```python
from build123d import *

# Parameters (mm, degrees)
PAD004_DEPTH    = 50
PAD003_DEPTH    = 50
BOX001_W        = 33
BOX001_H        = 20
BOX001_DEPTH    = 51
BOX_W           = 33
BOX_H           = 20
BOX_DEPTH       = 51
BOX002_W        = 33
BOX002_H        = 20
BOX002_DEPTH    = 51
BOX003_W        = 33
BOX003_H        = 20
BOX003_DEPTH    = 51
SKETCH_R        = 25
PAD_DEPTH       = 30
PAD002_DEPTH    = 50
SKETCH001_R     = 40
PAD001_DEPTH    = 75
SKETCH005_W     = 21.319589
SKETCH005_H     = 49.375387
POCKET_DEPTH    = 0.2
SKETCH006_R     = 15
POCKET001_DEPTH = 43.555516


with BuildPart() as pad004:
    # Sketch004 → Pad004 (new body, symmetric)
    with BuildSketch(Plane.XZ):
        Polygon((-40, 70), (-20, 104.849875), (-40, 104.849875), align=None)
    extrude(amount=PAD004_DEPTH, both=True)


with BuildPart() as pad003:
    # Sketch003 → Pad003 (new body, symmetric)
    with BuildSketch(Plane.XZ):
        Polygon((20, 105), (40, 69.438118), (40, 105), align=None)
    extrude(amount=PAD003_DEPTH, both=True)


with BuildPart() as cubo001:
    # Box001 → Box001 (new body)
    with BuildSketch(Plane(origin=(5, -40, 55), x_dir=(1, 0, 0), z_dir=(0, 0, 1))):
        with Locations((16.5, 10)):
            Rectangle(BOX001_W, BOX001_H)
    extrude(amount=BOX001_DEPTH)


with BuildPart() as cubo:
    # Box → Box (new body)
    with BuildSketch(Plane(origin=(5, 20, 55), x_dir=(1, 0, 0), z_dir=(0, 0, 1))):
        with Locations((16.5, 10)):
            Rectangle(BOX_W, BOX_H)
    extrude(amount=BOX_DEPTH)


with BuildPart() as cubo002:
    # Box002 → Box002 (new body)
    with BuildSketch(Plane(origin=(-38, -40, 55), x_dir=(1, 0, 0), z_dir=(0, 0, 1))):
        with Locations((16.5, 10)):
            Rectangle(BOX002_W, BOX002_H)
    extrude(amount=BOX002_DEPTH)


with BuildPart() as cubo003:
    # Box003 → Box003 (new body)
    with BuildSketch(Plane(origin=(-38, 20, 55), x_dir=(1, 0, 0), z_dir=(0, 0, 1))):
        with Locations((16.5, 10)):
            Rectangle(BOX003_W, BOX003_H)
    extrude(amount=BOX003_DEPTH)


with BuildPart() as pad:
    # Sketch → Pad (new body)
    with BuildSketch(Plane.XY):
        Circle(SKETCH_R)
    extrude(amount=PAD_DEPTH)


with BuildPart() as pad002:
    # Sketch002 → Pad002 (new body, symmetric)
    with BuildSketch(Plane(origin=(-81, 0, 6), x_dir=(1, 0, 0), z_dir=(0, -1, 0))):
        with BuildLine():
            Line((61.374028, 37.554516), (102.260882, 37.554516))
            Line((102.260882, 37.554516), (102.260882, 66.257331))
            ThreePointArc((102.260882, 66.257331), (98.26163, 79.156523), (87.211113, 86.919851))
            Line((87.211113, 86.919851), (87.11186, 102.554516))
            Line((87.11186, 102.554516), (75.11186, 102.554516))
            Line((75.11186, 102.554516), (75.158353, 85.860966))
            ThreePointArc((75.158353, 85.860966), (65.381997, 78.874221), (61.374028, 67.54603))
            Line((61.374028, 37.554516), (61.374028, 67.54603))
        make_face()
    extrude(amount=PAD002_DEPTH, both=True)


with BuildPart() as pocket001:
    # Pad001 base: copy of Pad
    add(pad.part)

    # Sketch001 → Pad001 (new body)
    with BuildSketch(Plane.XY.offset(30)):
        Circle(SKETCH001_R)
    extrude(amount=PAD001_DEPTH)

    # Cut: cut Pad002
    add(pad002.part, mode=Mode.SUBTRACT)

    # Fusion: union Pad
    add(pad.part)

    # Cut001: cut Cubo003
    add(cubo003.part, mode=Mode.SUBTRACT)

    # Cut002: cut Cubo002
    add(cubo002.part, mode=Mode.SUBTRACT)

    # Cut003: cut Cubo
    add(cubo.part, mode=Mode.SUBTRACT)

    # Cut004: cut Cubo001
    add(cubo001.part, mode=Mode.SUBTRACT)

    # Cut005: cut Pad003
    add(pad003.part, mode=Mode.SUBTRACT)

    # Cut006: cut Pad004
    add(pad004.part, mode=Mode.SUBTRACT)

    # Sketch005 → Pocket (cut)
    with BuildSketch(Plane.XY.offset(105)):
        with Locations((-30.63901, -1.115778)):
            Rectangle(SKETCH005_W, SKETCH005_H)
    extrude(amount=-POCKET_DEPTH, mode=Mode.SUBTRACT)

    # Sketch006 → Pocket001 (cut, through all)
    with BuildSketch(Plane.XY.offset(43.554516)):
        Circle(SKETCH006_R)
    extrude(amount=-POCKET001_DEPTH, mode=Mode.SUBTRACT)


solid = pocket001.part
```
Model file for the job. Use its own axes, mm. A direction names the side the tool comes from. Round coordinates to 2 decimals unless told otherwise and drop trailing zeros. Write each loop counter-clockwise with the first axis right and the second up, starting at its lowest first coordinate (ties: lowest second). Pieces come first, ordered by that corner, then holes. Notation, with made-up numbers: (17, -32.75) - (22, -32.75) arc R5 ccw to (22, -23.75) - close; hole circle Ø5 at (10.25, 30.5). An arc over 180 degrees is marked (long way). One line per item, written item: value.
(1) Cut at C-C, the plane x = 0. Give the cut face in (y, z).
Values follow:
outline: (-40, 30) - (-25, 30) - (-25, 0) - (-15, 0) - (-15, 43.55) - (-40, 43.55) - close; (15, 0) - (25, 0) - (25, 30) - (40, 30) - (40, 43.55) - (15, 43.55) - close
(2) Cut at D-D, the plane x = 17. Give the cut face in (y, z).
Values follow:
outline: (-36.21, 30) - (-18.33, 30) - (-18.33, 0) - (18.33, 0) - (18.33, 30) - (36.21, 30) - (36.21, 43.55) - (-36.21, 43.55) - close; (-20, 85.51) - (20, 85.51) - (20, 105) - (-20, 105) - close
(3) Drop flat-ended pins along their axis: P1, Ø15, axis at y = 10, z = 61, coming from the +X side; P2, Ø14.5, axis at y = -14.5, z = 64.5, coming from the -X side; P3, Ø23, axis at x = -21.5, z = 83.5, coming from the -Y side. Give the stop position or say it passes through.
Values follow:
P1: stops at x = 39.92
P2: stops at x = -39.34
P3: stops at y = -20
(4) Two-plate mould, pull along Y, no slides. Class faces 1 (the flat face through (23, -20, 80)), 2 (the cylindrical face through (-14.985, 0.66, 22.082)), 3 (the cylindrical face through (-15.515, -0.28, 85.01)): pulls with the +Y half, pulls with the -Y half, needs draft (parallel to the pull), parting line crosses it, or undercut.
Values follow:
face 1: pulls with the -Y half
face 2: undercut
face 3: needs draft
(5) Cut at A-A, the plane y = 0. Give the cut face in (x, z).
Values follow:
outline: (-40, 30) - (-25, 30) - (-25, 0) - (-15, 0) - (-15, 43.55) - (-19.63, 43.55) - (-19.63, 73.55) arc R20 cw to (-5.84, 91.86) - (-5.88, 105) - (-19.98, 105) - (-19.98, 104.8) - (-20.03, 104.8) - (-40, 70) - close; (6.13, 105) - (6.21, 92.92) arc R20.91 cw to (21.26, 72.26) - (21.26, 43.55) - (15, 43.55) - (15, 0) - (25, 0) - (25, 30) - (40, 30) - (40, 69.44) - (20, 105) - close
(6) Wall check: probe 1 along Y at (x, z) = (0, 22); probe 2 along Z at (x, y) = (-24.5, 26); probe 3 along X at (y, z) = (7.5, 79). Give the ranges that are in metal, low to high.
Values follow:
probe 1: y = -25 to -15, 15 to 25
probe 2: z = 30 to 55
probe 3: x = -34.83 to -18.67, 20.34 to 34.62
(7) 3-axis set-ups, long thin cutter, end or side, ignore diameter. For faces 4 (the flat face through (21.261, 0, 55)), 5 (the flat face through (-24, -20, 80)), 6 (the flat face through (17.22, 18.34, 30)), 7 (the flat face through (23, 20, 80)): which of +Z, -Z, +X, -X, +Y, -Y reach the whole face in a straight line?
Values follow:
face 4: +Y, -Y
face 5: +Z, +X, -X, -Y
face 6: -Z
face 7: +Z, +X, -X, +Y
(8) Cut at B-B, the plane z = 58. Give the cut face in (x, y).
Values follow:
outline: (-34.64, -20) - (-19.63, -20) - (-19.63, 20) - (-34.64, 20) arc R40 ccw to start; (21.26, -20) - (34.64, -20) arc R40 ccw to (34.64, 20) - (21.26, 20) - close
